from build123d import *

# Parameters (mm, degrees)
SKETCH1_W             = 12.7
SKETCH1_H             = 28.448
BOSS_EXTRUDE1_DEPTH   = 19.05
SKETCH2_W             = 12.7
SKETCH2_H             = 12.7
CUT_EXTRUDE1_DEPTH    = 27.953936188
SKETCH5_R             = 1.5875
CUT_EXTRUDE2_DEPTH    = 35.82116747
F_4_40_TAPPED_HOLE1_D = 2.2606


with BuildPart() as part:
    # Sketch1 → Boss-Extrude1 (new body)
    with BuildSketch(Plane(origin=(0, 0, 0), x_dir=(1, 0, 0), z_dir=(0, 1, 0))):
        Rectangle(SKETCH1_W, SKETCH1_H)
    extrude(amount=BOSS_EXTRUDE1_DEPTH)

    # Sketch2 → Cut-Extrude1 (cut, through all)
    with BuildSketch(Plane(origin=(6.35, 0, 0), x_dir=(0, 0, -1), z_dir=(1, 0, 0))):
        with Locations((0, 12.7)):
            Rectangle(SKETCH2_W, SKETCH2_H)
    extrude(amount=-CUT_EXTRUDE1_DEPTH, mode=Mode.SUBTRACT)

    # Sketch5 → Cut-Extrude2 (cut, through all)
    with BuildSketch(Plane.XY.offset(14.224)):
        with Locations((0, 15.875)):
            Circle(SKETCH5_R)
    extrude(amount=-CUT_EXTRUDE2_DEPTH, mode=Mode.SUBTRACT)

    # #4-40 Tapped Hole1 (through all)
    with Locations(Plane(origin=(0, 0, 0), x_dir=(-1, 0, 0), z_dir=(0, -1, 0))):
        with Locations((0, 0)):
            Hole(F_4_40_TAPPED_HOLE1_D / 2)


solid = part.part
Model file for the job. Use its own axes, mm. A direction names the side the tool comes from. Coordinates: 2 decimals unless noted, no trailing zeros. Write each loop counter-clockwise with the first axis right and the second up, starting at its lowest first coordinate (ties: lowest second). Pieces come first, ordered by that corner, then holes. Notation, with made-up numbers: (14.25, 49.25) -> (69.25, 49.25) arc R28 ccw to (69.25, 68.25) -> close; hole circle Ø10 at (81.5, 25). An arc over 180 degrees is marked (long way). One line per item, written item: value. Start each with the question number.
1) Pull direction Z, two halves, no side cores. Call faces 3 (the face through (0, 13, -6.35)), 4 (the face through (0.1, 6.35, -1.3)), 5 (the face through (0, 9, 14.224)), 6 (the face through (0, 19.05, 10)): +Z half, -Z half, draft (parallel to the pull), parting line (faces both ways), or undercut.
2) Which spindle directions (+Z, -Z, +X, -X, +Y, -Y) get a long thin tool onto all of the face, cutting with end or side? Do faces 1 (the face through (-0.344, 14.325, -10.232)), 2 (the face through (0, 13, 6.35)). Say none if no direction does.
3) Probe probe 1 along Y at (x, z) = (0, 12.75); probe 2 along Z at (x, y) = (-1, 17.25). List the from-to ranges inside material, lowest first.
4) Slice it at B-B on x = 0. Write the cut outline in (y, z), then the cut area to 3 significant figures.
5) Slice it at A-A on y = 13.5. Write the cut outline in (x, z), then the cut area to 3 significant figures.
6) Slice it at C-C on z = 0. Write the cut outline in (x, y), then the cut area to 3 significant figures.
7) Slice it at D-D on x = -3.25. Write the cut outline in (y, z).
8) Flat gauge pins, fed straight in: pin 1 Ø1.4 at (x, z) = (0, 0) entering from +Y; pin 2 Ø4 at (x, z) = (3, 0) entering from +Y. Where does each tip first touch, or does it go through?
Answers follow:
1. face 3: undercut
1. face 4: undercut
1. face 5: +Z half
1. face 6: draft
2. face 1: +Z, -Z
2. face 2: +X, -X, +Y
3. probe 1: 0 to 14.29, 17.46 to 19.05
3. probe 2: -14.22 to -6.35, 6.35 to 14.22
4. outline: (0, -14.22) -> (14.29, -14.22) -> (14.29, -6.35) -> (6.35, -6.35) -> (6.35, -1.13) -> (0, -1.13) -> close; (0, 1.13) -> (6.35, 1.13) -> (6.35, 6.35) -> (14.29, 6.35) -> (14.29, 14.22) -> (0, 14.22) -> close; (17.46, -14.22) -> (19.05, -14.22) -> (19.05, -6.35) -> (17.46, -6.35) -> close; (17.46, 6.35) -> (19.05, 6.35) -> (19.05, 14.22) -> (17.46, 14.22) -> close
4. area: 316 mm2
5. outline: (-6.35, -14.22) -> (6.35, -14.22) -> (6.35, -6.35) -> (-6.35, -6.35) -> close; (-6.35, 6.35) -> (6.35, 6.35) -> (6.35, 14.22) -> (-6.35, 14.22) -> close
5. area: 200 mm2
6. outline: (-6.35, 0) -> (-1.13, 0) -> (-1.13, 6.35) -> (-6.35, 6.35) -> close; (1.13, 0) -> (6.35, 0) -> (6.35, 6.35) -> (1.13, 6.35) -> close
6. area: 66.3 mm2
7. outline: (0, -14.22) -> (19.05, -14.22) -> (19.05, -6.35) -> (6.35, -6.35) -> (6.35, 6.35) -> (19.05, 6.35) -> (19.05, 14.22) -> (0, 14.22) -> close
8. pin 1: through
8. pin 2: y = 6.35
